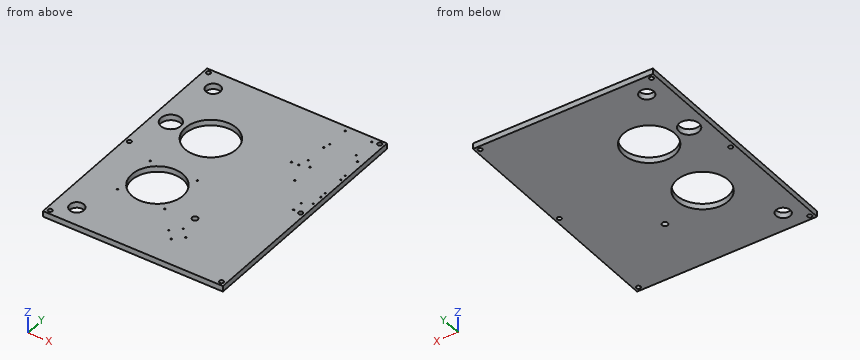
```python
from build123d import *

# Parameters (mm, degrees)
SKETCH2_W           = 400.05
SKETCH2_H           = 527.05
SKETCH2_R           = 4.7625
BOSS_EXTRUDE1_DEPTH = 12.7
SKETCH3_R           = 15.875
SKETCH3_R_2         = 22.225
SKETCH3_R_3         = 57.15
CUT_EXTRUDE1_DEPTH  = 332.084152822
SKETCH4_R           = 1.5875
CUT_EXTRUDE2_DEPTH  = 1.5875
SKETCH7_R           = 6.35
CUT_EXTRUDE4_DEPTH  = 332.084152822


with BuildPart() as part:
    # Sketch2 → Boss-Extrude1 (new body)
    with BuildSketch(Plane.XY):
        Rectangle(SKETCH2_W, SKETCH2_H)
        with Locations((-190.5, 254)):
            Circle(SKETCH2_R, mode=Mode.SUBTRACT)
        with Locations((190.5, 254)):
            Circle(SKETCH2_R, mode=Mode.SUBTRACT)
        with Locations((-190.5, -254)):
            Circle(SKETCH2_R, mode=Mode.SUBTRACT)
        with Locations((190.5, -254)):
            Circle(SKETCH2_R, mode=Mode.SUBTRACT)
        with Locations((-190.5, 0)):
            Circle(SKETCH2_R, mode=Mode.SUBTRACT)
        with Locations((190.5, 0)):
            Circle(SKETCH2_R, mode=Mode.SUBTRACT)
    extrude(amount=BOSS_EXTRUDE1_DEPTH)

    # Sketch3 → Cut-Extrude1 (cut, through all)
    with BuildSketch(Plane.XY.offset(12.7)):
        with Locations((-155.575, 219.075)):
            Circle(SKETCH3_R)
        with Locations((-161.925, 92.075)):
            Circle(SKETCH3_R_2)
        with Locations((-73.025, 92.075)):
            Circle(SKETCH3_R_3)
        with Locations((-73.025, -79.375)):
            Circle(SKETCH3_R_3)
        with Locations((-155.575, -219.075)):
            Circle(SKETCH3_R)
    extrude(amount=-CUT_EXTRUDE1_DEPTH, mode=Mode.SUBTRACT)

    # Sketch4 → Cut-Extrude2 (cut)
    with BuildSketch(Plane.XY.offset(12.7)):
        with Locations((60.325, -180.975)):
            Circle(SKETCH4_R)
        with Locations((22.225, -180.975)):
            Circle(SKETCH4_R)
        with Locations((41.275, -161.925)):
            Circle(SKETCH4_R)
        with Locations((193.675, 35.71875)):
            Circle(SKETCH4_R)
        with Locations((174.625, 0)):
            Circle(SKETCH4_R)
        with Locations((193.675, 60.325)):
            Circle(SKETCH4_R)
        with Locations((193.675, 74.6125)):
            Circle(SKETCH4_R)
        with Locations((193.675, 123.825)):
            Circle(SKETCH4_R)
        with Locations((125.4125, 123.825)):
            Circle(SKETCH4_R)
        with Locations((125.4125, 74.6125)):
            Circle(SKETCH4_R)
        with Locations((88.9, 117.475)):
            Circle(SKETCH4_R)
        with Locations((104.775, 117.475)):
            Circle(SKETCH4_R)
        with Locations((115.8875, 250.825)):
            Circle(SKETCH4_R)
        with Locations((174.625, 250.825)):
            Circle(SKETCH4_R)
        with Locations((174.625, 201.6125)):
            Circle(SKETCH4_R)
        with Locations((115.8875, 201.6125)):
            Circle(SKETCH4_R)
        with Locations((112.395, 187.325)):
            Circle(SKETCH4_R)
        with Locations((187.325, 187.325)):
            Circle(SKETCH4_R)
        with Locations((111.125, 139.065)):
            Circle(SKETCH4_R)
        with Locations((193.675, 139.065)):
            Circle(SKETCH4_R)
        with Locations((41.275, -200.025)):
            Circle(SKETCH4_R)
        with Locations((174.625, 24.60625)):
            Circle(SKETCH4_R)
        with Locations((-125.4125, -26.9875)):
            Circle(SKETCH4_R)
        with Locations((-20.6375, -26.9875)):
            Circle(SKETCH4_R)
        with Locations((-20.6375, -131.7625)):
            Circle(SKETCH4_R)
        with Locations((-125.4125, -131.7625)):
            Circle(SKETCH4_R)
    extrude(amount=-CUT_EXTRUDE2_DEPTH, mode=Mode.SUBTRACT)

    # Sketch7 → Cut-Extrude4 (cut, through all)
    with BuildSketch(Plane.XY.offset(12.7)):
        with Locations((41.275, -123.825)):
            Circle(SKETCH7_R)
    extrude(amount=-CUT_EXTRUDE4_DEPTH, mode=Mode.SUBTRACT)


solid = part.part
```
Can you work these out from the model? Positions are in its coordinate system, mm. Round coordinates to 2 decimals unless told otherwise and drop trailing zeros. Loops run counter-clockwise (first coordinate to the right, second up) from the corner with the lowest first, then second, coordinate; pieces in that order, holes last. Notation, with made-up numbers: (-13, -39.5) -> (40, -39.5) arc R23 ccw to (40, -13.5) -> close; hole circle Ø7 at (82, 82.5). An arc over 180 degrees is marked (long way). Answer in a Markdown table with one row per item.
Item 1: Suppose I cut it at B-B, the plane z = 8.75. Give the number of separate pieces and of enclosed holes in the cut face, plus the area to 3 significant figures.
Answer block:
| item | result |
|---|---|
| separate pieces | 1 |
| enclosed holes | 12 |
| area | 187,000 mm² |
Item 2: Suppose I cut it at A-A, the plane y = -209. List the corners of the cut face in (x, z) for me (3 decimals), plus the area to 3 significant figures.
Answer block:
| item | result |
|---|---|
| outline | (-200.025, 0) -> (-167.843, 0) -> (-167.843, 12.7) -> (-200.025, 12.7) -> close; (-143.307, 0) -> (200.025, 0) -> (200.025, 12.7) -> (-143.307, 12.7) -> close |
| area | 4,770 mm² |
Item 3: Will these pins go through, and if not, where does the flat tip stop? P1, Ø1.9, axis at x = 115.89, y = 201.61, coming from the -Z side; P2, Ø1.6, axis at x = 125, y = 124, coming from the +Z side; P3, Ø5.5, axis at x = 190.5, y = -254, coming from the +Z side.
Answer block:
| item | result |
|---|---|
| P1 | z = 0 |
| P2 | z = 11.11 |
| P3 | through |
Item 4: If I drill on probe 1 along Y at (x, z) = (-122.5, 2.25) (3 decimals); probe 2 along Y at (x, z) = (-28.5, 9.75) (3 decimals); probe 3 along Y at (x, z) = (-150, 6.75) (3 decimals), over which ranges is the centre line in solid material (lowest first)?
Answer block:
| item | result |
|---|---|
| probe 1 | -263.525 to -107.982, -50.768 to 63.468, 120.682 to 263.525 |
| probe 2 | -263.525 to -115.203, -43.547 to 56.247, 127.903 to 263.525 |
| probe 3 | -263.525 to -233.939, -204.211 to 73.32, 110.83 to 204.211, 233.939 to 263.525 |
